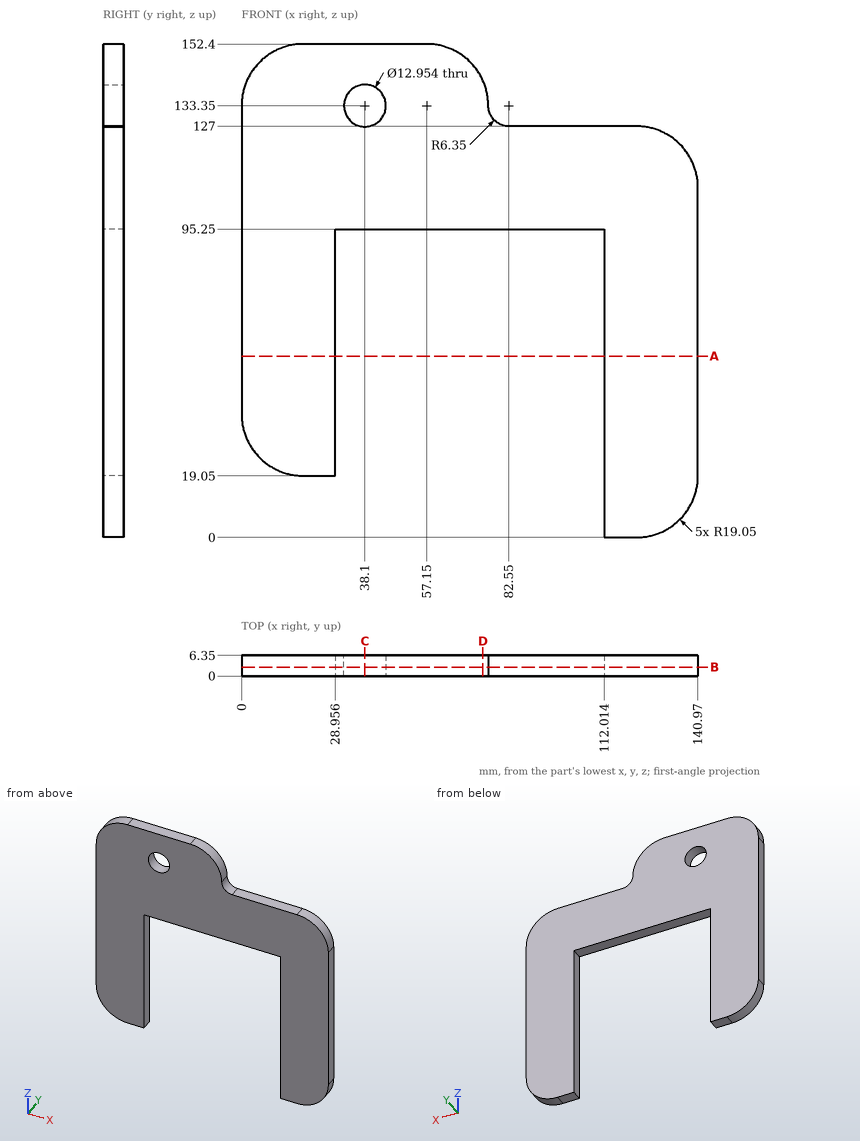
Print and shaded views of the part. All mm, measured from the part's lowest x, y and z. Give positions to 0.01 mm unless a question says otherwise; leave off trailing zeros. Loops run counter-clockwise (first coordinate to the right, second up) from the corner with the lowest first, then second, coordinate; pieces in that order, holes last. Notation, with made-up numbers: (-35, 59.25) - (-19, 59.25) arc R23 cw to (-19, 91.25) - close; hole circle Ø9 at (20, 74). An arc over 180 degrees is marked (long way). One line per item, written item: value. Start each with the question number.
1. Slice it at B-B (y = 2.75). List the corners of the cut face in (x, z), plus the area to 3 significant figures.
2. Slice it at A-A (z = 56). List the corners of the cut face in (x, y).
3. Probe L1, parallel to X at y = 3.25, z = 60; L2, parallel to Z at x = 38.1, y = 3.25; L3, parallel to X at y = 1.5, z = 133. List the from-to ranges inside material, lowest first. Write a range as from..to.
4. Pin check, flat tips, straight feed: pin 1 (12 mm diameter, centred on x = 40.5, z = 19, fed in from +Y); pin 2 (1.9 mm diameter, centred on x = 97, y = 3.5, fed in from +Z); pin 3 (20.5 mm diameter, centred on x = 38.1, z = 133.35, fed in from -Y); pin 4 (1.9 mm diameter, centred on x = 26, y = 3, fed in from -Z). Stop position of each tip, or through.
5. Slice it at D-D (x = 74.5). List the corners of the cut face in (y, z), plus the area to 3 significant figures.
6. Slice it at C-C (x = 38.1). List the corners of the cut face in (y, z).
Solution:
1. outline: (0, 38.1) arc R19.05 ccw to (19.05, 19.05) - (28.96, 19.05) - (28.96, 95.25) - (112.01, 95.25) - (112.01, 0) - (121.92, 0) arc R19.05 ccw to (140.97, 19.05) - (140.97, 107.95) arc R19.05 ccw to (121.92, 127) - (82.55, 127) arc R6.35 cw to (76.2, 133.35) arc R19.05 ccw to (57.15, 152.4) - (19.05, 152.4) arc R19.05 ccw to (0, 133.35) - close; hole circle Ø12.95 at (38.1, 133.35)
1. area: 10,900 mm^2
2. outline: (0, 0) - (28.96, 0) - (28.96, 6.35) - (0, 6.35) - close; (112.01, 0) - (140.97, 0) - (140.97, 6.35) - (112.01, 6.35) - close
3. L1: x = 0..28.96, 112.01..140.97
3. L2: z = 95.25..126.87, 139.83..152.4
3. L3: x = 0..31.63, 44.57..76.21
4. pin 1: passes through
4. pin 2: stops at z = 127
4. pin 3: stops at y = 0
4. pin 4: stops at z = 19.05
5. outline: (0, 95.25) - (6.35, 95.25) - (6.35, 141.22) - (0, 141.22) - close
5. area: 292 mm^2
6. outline: (0, 95.25) - (6.35, 95.25) - (6.35, 126.87) - (0, 126.87) - close; (0, 139.83) - (6.35, 139.83) - (6.35, 152.4) - (0, 152.4) - close
